Design review of the part built by this model. Coordinates are the model's own, in mm. Coordinates: 2 decimals unless noted, no trailing zeros. Order: outer loops, then holes, each group sorted by start corner. A loop starts at its lowest first (then second) coordinate and runs counter-clockwise, first axis right, second up. Notation, with made-up numbers: (38, 69.25) -> (60, 69.25) arc R26 ccw to (60, 92.25) -> close; hole circle Ø10 at (47, -3.5). An arc over 180 degrees is marked (long way). Use a Markdown table: item, result. Add a question column.
Q1. Add section C-C (z = -84.25). State the section outline as (x, y) points.
Q2. Wall thickness on probe 1 along Y at (x, z) = (1.5, -84.25); probe 2 along Y at (x, z) = (0.75, 0.5); probe 3 along Y at (x, z) = (0.25, 20.5): over which ranges is each line inside the solid? List them lowest first.
Q3. Add section A-A (z = 0). State the section outline as (x, y) points, then the cut area to 3 significant figures.
Q4. Insertion check: pin 1 (4 mm diameter, centred on y = 15, z = -84.25, fed in from -X); pin 2 (1 mm diameter, centred on x = 1.5, z = -78.5, fed in from +Y); pin 3 (0.6 mm diameter, centred on x = 1, z = -35, fed in from -Y). Each pin has a flat end and moves straight along its axis. Give the tip position at first contact, or say it passes through.
Q5. Add section D-D (x = 0.95). Count the separate pieces of the cut face and the enclosed holes in it, then the cut area to 3 significant figures.
Q6. Add section B-B (y = 0). State the section outline as (x, z) points, then the cut area to 3 significant figures.
Autodesk Inventor part; units mm, degrees
ref_plane "YZ Plane" through (0, 0, 0) normal (1, 0, 0) x (0, 1, 0)
ref_plane "XZ Plane" through (0, 0, 0) normal (0, 1, 0) x (-1, 0, 0)
ref_plane "XY Plane" through (0, 0, 0) normal (0, 0, 1) x (1, 0, 0)
sketch "スケッチ1" plane through (0, 0, 0) normal (1, 0, 0) x (0, 1, 0)
  circle A0 centre (0, 0) radius 39.25
  circle A1 centre (0, 0) radius 33
  line L0 (8, 0) -> (-8, 0)
  line L1 (-8, 0) -> (-8, -36)
  line L2 (-8, -36) -> (8, -36)
  line L3 (8, -36) -> (8, 0)
  line L4 (30, -39.25) -> (-30, -39.25)
  line L5 (-30, -39.25) -> (-30, -99.25)
  line L6 (-30, -99.25) -> (30, -99.25)
  line L7 (30, -99.25) -> (30, -39.25)
  line L8 (30, -39.25) -> (37.874, -10.3018)
  line L9 (-30, -39.25) -> (-37.874, -10.3018)
  point P0 (8, 32.0156)
  point P1 (8, -32.0156)
  point P2 (-8, -32.0156)
  point P3 (-8, 32.0156)
  point P4 (0, -39.25)
  dimension "d0" = 78.5
  dimension "d1" = 66
  dimension "d2" = 16
  dimension "d3" = 36
  dimension "d4" = 8
  dimension "d5" = 0
  dimension "d6" = 60
  dimension "d7" = 60
  dimension "d8" = 30
  dimension "d9" = 39.25
extrude "押し出し1" add sketch "スケッチ1" along normal blind 2
sketch "スケッチ2" plane through (2, 0, 0) normal (1, 0, 0) x (0, 0, -1)
  circle A0 centre (0, 0) radius 36.5
  point P0 (-36.5, 0)
  point P1 (-27.9606, -23.4617)
  point P2 (-6.3382, -35.9455)
  point P3 (18.25, -31.6099)
  point P4 (34.2988, -12.4837)
  point P5 (34.2988, 12.4837)
  point P6 (18.25, 31.6099)
  point P7 (-6.3382, 35.9455)
  point P8 (-27.9606, 23.4617)
  dimension "d12" = 73
  dimension "d15" = 360
hole "穴1" at (2, 0, 36.5) at (2, -23.4617, 27.9606) at (2, -35.9455, 6.3382) at (2, -31.6099, -18.25) at (2, -12.4837, -34.2988) at (2, 12.4837, -34.2988) at (2, 31.6099, -18.25) at (2, 35.9455, 6.3382) at (2, 23.4617, 27.9606) direction (-1, 0, 0) diameter 3.2 end through all
sketch "スケッチ3" plane through (2, 0, 0) normal (1, 0, 0) x (0, 0, -1)
  line L0 (54.25, 15) -> (84.25, 15)
  line L1 (84.25, 15) -> (84.25, -15)
  line L2 (84.25, -15) -> (54.25, -15)
  line L3 (54.25, -15) -> (54.25, 15)
  line L4 (99.25, -30) -> (99.25, 30)
  point P0 (0, 0)
  dimension "d24" = 30
  dimension "d25" = 30
  dimension "d26" = 15
  dimension "d27" = 15
hole "穴2" at (2, 15, -54.25) at (2, -15, -54.25) at (2, 15, -84.25) at (2, -15, -84.25) direction (-1, 0, 0) diameter 4.2 end through all
properties part number "link3_plate2" material "アルミニウム 6061"
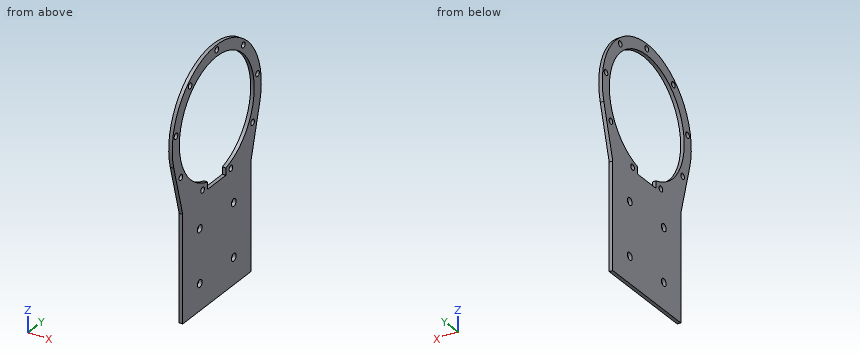
Established:
| question | item | result |
|---|---|---|
| 1 | outline | (0, -30) -> (2, -30) -> (2, -17.1) -> (0, -17.1) -> close; (0, -12.9) -> (2, -12.9) -> (2, 12.9) -> (0, 12.9) -> close; (0, 17.1) -> (2, 17.1) -> (2, 30) -> (0, 30) -> close |
| 2 | probe 1 | -30 to -17.1, -12.9 to 12.9, 17.1 to 30 |
| 2 | probe 2 | -39.25 to -33, 33 to 39.25 |
| 2 | probe 3 | -33.47 to -25.86, 25.86 to 33.47 |
| 3 | outline | (0, -39.25) -> (2, -39.25) -> (2, -33) -> (0, -33) -> close; (0, 33) -> (2, 33) -> (2, 39.25) -> (0, 39.25) -> close |
| 3 | area | 25.0 mm^2 |
| 4 | pin 1 | through |
| 4 | pin 2 | y = 30 |
| 4 | pin 3 | y = -31.24 |
| 5 | separate pieces | 1 |
| 5 | enclosed holes | 14 |
| 5 | area | 5,180 mm^2 |
| 6 | outline | (0, -99.25) -> (2, -99.25) -> (2, -36) -> (0, -36) -> close; (0, 33) -> (2, 33) -> (2, 34.9) -> (0, 34.9) -> close; (0, 38.1) -> (2, 38.1) -> (2, 39.25) -> (0, 39.25) -> close |
| 6 | area | 133 mm^2 |
